Input: dimensioned drawing with shaded views. Units: mm. Origin: part minimum x, y, z. A direction names the side the tool comes from. Round coordinates to 2 decimals unless told otherwise and drop trailing zeros. Loops run counter-clockwise (first coordinate to the right, second up) from the corner with the lowest first, then second, coordinate; pieces in that order, holes last. Notation, with made-up numbers: M 32,23 L 61,23 A20 ccw 61,33 Z; hole C -23,74.5 d11. An arc over 180 degrees is marked long. One line per item, written item: value.
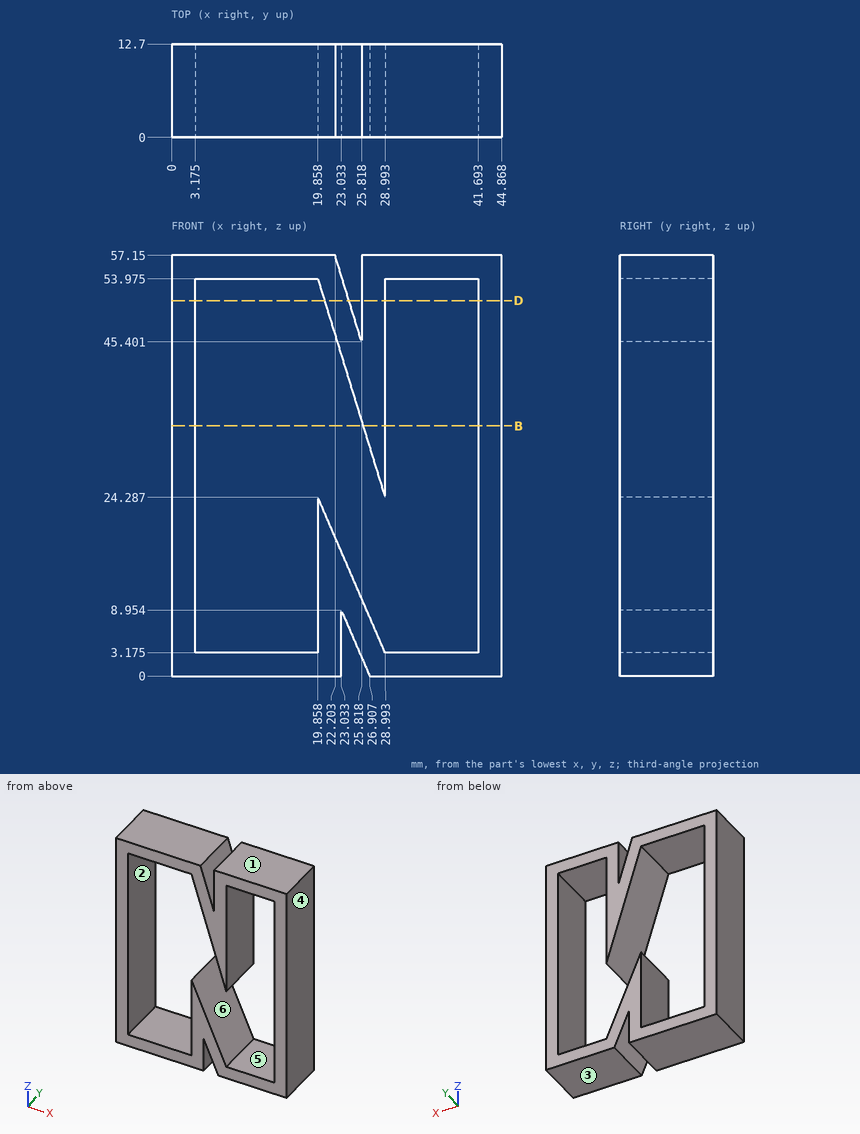
1. Ray query, line 1 (X direction, y = 8.75, z = 27) (1 decimal); line 2 (X direction, y = 3.25, z = 18) (1 decimal); line 3 (X direction, y = 2.75, z = 49) (1 decimal). Return the intervals inside material, ascending. Write a range as [from, to].
Report:
line 1: x = [0, 3.2], [28.2, 29], [41.7, 44.9]
line 2: x = [0, 3.2], [19.9, 22.6], [41.7, 44.9]
line 3: x = [0, 3.2], [21.4, 24.7], [25.8, 29], [41.7, 44.9]
2. Section query B-B (z = 34). Return the cut outline in (x, y) (1 decimal).
Report:
outline: M 0,0 L 3.2,0 L 3.2,12.7 L 0,12.7 Z; M 26,0 L 29,0 L 29,12.7 L 26,12.7 Z; M 41.7,0 L 44.9,0 L 44.9,12.7 L 41.7,12.7 Z
3. Section query D-D (z = 51). Return the cut outline in (x, y) (1 decimal).
Report:
outline: M 0,0 L 3.2,0 L 3.2,12.7 L 0,12.7 Z; M 20.8,0 L 24.1,0 L 24.1,12.7 L 20.8,12.7 Z; M 25.8,0 L 29,0 L 29,12.7 L 25.8,12.7 Z; M 41.7,0 L 44.9,0 L 44.9,12.7 L 41.7,12.7 Z
4. Pull-direction query (X, two-part tool) for the marked faces 3, 4, 5 and 6; classes: released by +X, released by -X, zero draft, split by the parting line, or undercut.
Report:
face 3: zero draft
face 4: released by +X
face 5: undercut
face 6: undercut
5. Reachability of the marked faces 1 and 2 from +Z, -Z, +X, -X, +Y, -Y: full face, straight path, thin tool, end or side. Return the list, or none.
Report:
face 1: +Z, +X, -X, +Y, -Y
face 2: +Y, -Y
